```python
from build123d import *

# Parameters (mm, degrees)
F0_W     = 182.88
F0_H     = 127
F1_DEPTH = 25.4


with BuildPart() as f1:
    # F0 (on Top) → F1 (new body)
    with BuildSketch(Plane.XY):
        with BuildLine():
            ThreePointArc((-101.6, 68.961), (-104.4736819587, 75.8986819587), (-97.536, 73.025))
            Line((-97.536, 73.025), (-93.8328908066, 73.025))
            ThreePointArc((-93.8328908066, 73.025), (-107.0921755809, 78.5171755809), (-101.6, 65.2578908066))
            Line((-101.6, 65.2578908066), (-101.6, 68.961))
        make_face()
        with BuildLine():
            Line((-93.8328908066, 73.025), (-97.536, 73.025))
            ThreePointArc((-97.536, 73.025), (-98.7263180413, 70.1513180413), (-101.6, 68.961))
            Line((-101.6, 68.961), (-101.6, 65.2578908066))
            ThreePointArc((-101.6, 65.2578908066), (-96.1078244191, 67.5328244191), (-93.8328908066, 73.025))
        make_face()
        with BuildLine():
            Line((-7.7671091934, 73.025), (-93.8328908066, 73.025))
            ThreePointArc((-93.8328908066, 73.025), (-96.1078244191, 67.5328244191), (-101.6, 65.2578908066))
            Line((-101.6, 65.2578908066), (-101.6, 7.7671091934))
            ThreePointArc((-101.6, 7.7671091934), (-96.1078244191, 5.4921755809), (-93.8328908066, 0))
            ThreePointArc((-93.8328908066, 0), (-96.1078244191, -5.4921755809), (-101.6, -7.7671091934))
            Line((-101.6, -7.7671091934), (-101.6, -65.2578908066))
            ThreePointArc((-101.6, -65.2578908066), (-96.1078244191, -67.5328244191), (-93.8328908066, -73.025))
            Line((-93.8328908066, -73.025), (-7.7671091934, -73.025))
            ThreePointArc((-7.7671091934, -73.025), (0, -65.2578908066), (7.7671091934, -73.025))
            Line((7.7671091934, -73.025), (93.8328908066, -73.025))
            ThreePointArc((93.8328908066, -73.025), (96.1078244191, -67.5328244191), (101.6, -65.2578908066))
            Line((101.6, -65.2578908066), (101.6, -7.7671091934))
            ThreePointArc((101.6, -7.7671091934), (93.8328908066, 0), (101.6, 7.7671091934))
            Line((101.6, 7.7671091934), (101.6, 65.2578908066))
            ThreePointArc((101.6, 65.2578908066), (96.1078244191, 67.5328244191), (93.8328908066, 73.025))
            Line((93.8328908066, 73.025), (7.7671091934, 73.025))
            ThreePointArc((7.7671091934, 73.025), (0, 65.2578908066), (-7.7671091934, 73.025))
        make_face()
        Rectangle(F0_W, F0_H, mode=Mode.SUBTRACT)
        with BuildLine():
            ThreePointArc((7.7671091934, 73.025), (0, 80.7921091934), (-7.7671091934, 73.025))
            Line((-7.7671091934, 73.025), (-4.064, 73.025))
            ThreePointArc((-4.064, 73.025), (0, 77.089), (4.064, 73.025))
            Line((4.064, 73.025), (7.7671091934, 73.025))
        make_face()
        with BuildLine():
            Line((-4.064, 73.025), (-7.7671091934, 73.025))
            ThreePointArc((-7.7671091934, 73.025), (0, 65.2578908066), (7.7671091934, 73.025))
            Line((7.7671091934, 73.025), (4.064, 73.025))
            ThreePointArc((4.064, 73.025), (0, 68.961), (-4.064, 73.025))
        make_face()
        with BuildLine():
            ThreePointArc((-93.8328908066, 0), (-96.1078244191, 5.4921755809), (-101.6, 7.7671091934))
            Line((-101.6, 7.7671091934), (-101.6, 4.064))
            ThreePointArc((-101.6, 4.064), (-98.7263180413, 2.8736819587), (-97.536, 0))
            ThreePointArc((-97.536, 0), (-98.7263180413, -2.8736819587), (-101.6, -4.064))
            Line((-101.6, -4.064), (-101.6, -7.7671091934))
            ThreePointArc((-101.6, -7.7671091934), (-96.1078244191, -5.4921755809), (-93.8328908066, 0))
        make_face()
        with BuildLine():
            Line((-101.6, 4.064), (-101.6, 7.7671091934))
            ThreePointArc((-101.6, 7.7671091934), (-109.3671091934, 0), (-101.6, -7.7671091934))
            Line((-101.6, -7.7671091934), (-101.6, -4.064))
            ThreePointArc((-101.6, -4.064), (-105.664, 0), (-101.6, 4.064))
        make_face()
        with BuildLine():
            ThreePointArc((109.3671091934, 73.025), (101.6, 80.7921091934), (93.8328908066, 73.025))
            Line((93.8328908066, 73.025), (97.536, 73.025))
            ThreePointArc((97.536, 73.025), (101.6, 77.089), (105.664, 73.025))
            ThreePointArc((105.664, 73.025), (104.4736819587, 70.1513180413), (101.6, 68.961))
            Line((101.6, 68.961), (101.6, 65.2578908066))
            ThreePointArc((101.6, 65.2578908066), (107.0921755809, 67.5328244191), (109.3671091934, 73.025))
        make_face()
        with BuildLine():
            Line((97.536, 73.025), (93.8328908066, 73.025))
            ThreePointArc((93.8328908066, 73.025), (96.1078244191, 67.5328244191), (101.6, 65.2578908066))
            Line((101.6, 65.2578908066), (101.6, 68.961))
            ThreePointArc((101.6, 68.961), (98.7263180413, 70.1513180413), (97.536, 73.025))
        make_face()
        with BuildLine():
            ThreePointArc((-93.8328908066, -73.025), (-96.1078244191, -67.5328244191), (-101.6, -65.2578908066))
            Line((-101.6, -65.2578908066), (-101.6, -68.961))
            ThreePointArc((-101.6, -68.961), (-98.7263180413, -70.1513180413), (-97.536, -73.025))
            Line((-97.536, -73.025), (-93.8328908066, -73.025))
        make_face()
        with BuildLine():
            Line((-101.6, -68.961), (-101.6, -65.2578908066))
            ThreePointArc((-101.6, -65.2578908066), (-107.0921755809, -78.5171755809), (-93.8328908066, -73.025))
            Line((-93.8328908066, -73.025), (-97.536, -73.025))
            ThreePointArc((-97.536, -73.025), (-104.4736819587, -75.8986819587), (-101.6, -68.961))
        make_face()
        with BuildLine():
            ThreePointArc((109.3671091934, 0), (107.0921755809, 5.4921755809), (101.6, 7.7671091934))
            Line((101.6, 7.7671091934), (101.6, 4.064))
            ThreePointArc((101.6, 4.064), (104.4736819587, 2.8736819587), (105.664, 0))
            ThreePointArc((105.664, 0), (104.4736819587, -2.8736819587), (101.6, -4.064))
            Line((101.6, -4.064), (101.6, -7.7671091934))
            ThreePointArc((101.6, -7.7671091934), (107.0921755809, -5.4921755809), (109.3671091934, 0))
        make_face()
        with BuildLine():
            Line((101.6, 4.064), (101.6, 7.7671091934))
            ThreePointArc((101.6, 7.7671091934), (93.8328908066, 0), (101.6, -7.7671091934))
            Line((101.6, -7.7671091934), (101.6, -4.064))
            ThreePointArc((101.6, -4.064), (97.536, 0), (101.6, 4.064))
        make_face()
        with BuildLine():
            ThreePointArc((7.7671091934, -73.025), (0, -65.2578908066), (-7.7671091934, -73.025))
            Line((-7.7671091934, -73.025), (-4.064, -73.025))
            ThreePointArc((-4.064, -73.025), (0, -68.961), (4.064, -73.025))
            Line((4.064, -73.025), (7.7671091934, -73.025))
        make_face()
        with BuildLine():
            Line((-4.064, -73.025), (-7.7671091934, -73.025))
            ThreePointArc((-7.7671091934, -73.025), (0, -80.7921091934), (7.7671091934, -73.025))
            Line((7.7671091934, -73.025), (4.064, -73.025))
            ThreePointArc((4.064, -73.025), (0, -77.089), (-4.064, -73.025))
        make_face()
        with BuildLine():
            ThreePointArc((109.3671091934, -73.025), (107.0921755809, -67.5328244191), (101.6, -65.2578908066))
            Line((101.6, -65.2578908066), (101.6, -68.961))
            ThreePointArc((101.6, -68.961), (104.4736819587, -70.1513180413), (105.664, -73.025))
            ThreePointArc((105.664, -73.025), (101.6, -77.089), (97.536, -73.025))
            Line((97.536, -73.025), (93.8328908066, -73.025))
            ThreePointArc((93.8328908066, -73.025), (101.6, -80.7921091934), (109.3671091934, -73.025))
        make_face()
        with BuildLine():
            Line((101.6, -68.961), (101.6, -65.2578908066))
            ThreePointArc((101.6, -65.2578908066), (96.1078244191, -67.5328244191), (93.8328908066, -73.025))
            Line((93.8328908066, -73.025), (97.536, -73.025))
            ThreePointArc((97.536, -73.025), (98.7263180413, -70.1513180413), (101.6, -68.961))
        make_face()
    extrude(amount=F1_DEPTH)


solid = f1.part
```
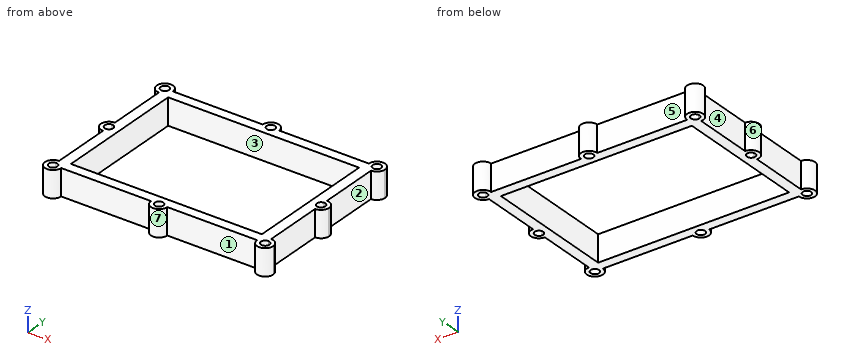
The listing builds one solid part. Answer for the finished solid, in the listing's coordinates (mm). Face numbers are marked on the shaded views. A direction names the side the tool comes from. Give positions to 0.01 mm unless a question says otherwise; leave off trailing zeros. Write each loop counter-clockwise with the first axis right and the second up, starting at its lowest first coordinate (ties: lowest second). Pieces come first, ordered by that corner, then holes. Notation, with made-up numbers: (51.25, -7.75) -> (76.25, -7.75) arc R23 cw to (76.25, 19.25) -> close; hole circle Ø4 at (72.25, 3). An arc over 180 degrees is marked (long way). Write item = value, one per line. Start each with the question number.
1) Which of the six approach directions +Z, -Z, +X, -X, +Y, -Y give full straight-line access (tool end or side, diameter ignored) to the marked faces 1, 2, 3 and 4?
2) The part is cut by section B-B, the plane y = -13. Determine the outline of the cut face in (x, z), and give its area (3 significant figures).
3) The part is cut by section C-C, the plane x = -68. Determine the outline of the cut face in (y, z) (3 decimals), and give its area (3 significant figures).
4) The part is cut by section D-D, the plane z = 18.5. Count the separate pieces of the cut face and the enclosed holes in it, and give its area (3 significant figures).
5) The part is cut by section A-A, the plane x = 0. Determine the outline of the cut face in (y, z).
6) Straight lines are drawn through the part: line 1 along Y through (x, z) = (0, 14.75); line 2 along Y through (x, z) = (86.5, 12.5) (3 decimals); line 3 along X through (y, z) = (-48, 10.5). For each, find the intervals that lie inside material, in ascending order.
7) Determine the mould class of the marked faces 5, 6 and 7 for opening direction Y: +Y half, -Y half, draft (parallel to the pull), parting line (faces both ways), or undercut.
8) Each of these flat-tipped pins is pushed along its axis until it touches: pin 1 (1 mm diameter, centred on x = -80, z = 18.5, fed in from +Y) (3 decimals); pin 2 (2 mm diameter, centred on y = -23, z = 5, fed in from +X); pin 3 (10 mm diameter, centred on x = 58.5, z = 3, fed in from -Y) (3 decimals); pin 4 (13 mm diameter, centred on x = -101.6, y = -73.025, fed in from +Z). Where does it stop, or does it pass through?
Solutions:
q1.face_1 = +Z, -Z, -Y
q1.face_2 = +Z, -Z, +X
q1.face_3 = +Z, -Z
q1.face_4 = +Z, -Z, -X
q2.outline = (-101.6, 0) -> (-91.44, 0) -> (-91.44, 25.4) -> (-101.6, 25.4) -> close; (91.44, 0) -> (101.6, 0) -> (101.6, 25.4) -> (91.44, 25.4) -> close
q2.area = 516 mm²
q3.outline = (-73.025, 0) -> (-63.5, 0) -> (-63.5, 25.4) -> (-73.025, 25.4) -> close; (63.5, 0) -> (73.025, 0) -> (73.025, 25.4) -> (63.5, 25.4) -> close
q3.area = 484 mm²
q4.separate_pieces = 1
q4.enclosed_holes = 9
q4.area = 6,980 mm²
q5.outline = (-80.79, 0) -> (-77.09, 0) -> (-77.09, 25.4) -> (-80.79, 25.4) -> close; (-68.96, 0) -> (-63.5, 0) -> (-63.5, 25.4) -> (-68.96, 25.4) -> close; (63.5, 0) -> (68.96, 0) -> (68.96, 25.4) -> (63.5, 25.4) -> close; (77.09, 0) -> (80.79, 0) -> (80.79, 25.4) -> (77.09, 25.4) -> close
q6.line_1 = -80.79 to -77.09, -68.96 to -63.5, 63.5 to 68.96, 77.09 to 80.79
q6.line_2 = -73.025 to -63.5, 63.5 to 73.025
q6.line_3 = -101.6 to -91.44, 91.44 to 101.6
q7.face_5 = +Y half
q7.face_6 = undercut
q7.face_7 = -Y half
q8.pin_1 = 73.025
q8.pin_2 = 101.6
q8.pin_3 = -73.025
q8.pin_4 = 25.4
